Could you check a few things on this model? Use its own coordinates, in mm. Face numbers are marked on the shaded views. A direction names the side the tool comes from. Coordinates: 2 decimals unless noted, no trailing zeros. Loops run counter-clockwise (first coordinate to the right, second up) from the corner with the lowest first, then second, coordinate; pieces in that order, holes last. Notation, with made-up numbers: (-1.5, 12) - (41.5, 12) arc R15 ccw to (41.5, 37) - close; hole circle Ø7 at (9, 6.25). An arc over 180 degrees is marked (long way). Use CSV: the item, a comma, the result in double quotes.
from build123d import *

# Parameters (mm, degrees)
F0_W     = 50
F0_H     = 50
F1_DEPTH = 60
F4_DEPTH = 50.001
F5_DEPTH = 50.001


with BuildPart() as f1:
    # F0 (on Top) → F1 (new body)
    with BuildSketch(Plane.XY):
        with Locations((25, 25)):
            Rectangle(F0_W, F0_H)
    extrude(amount=F1_DEPTH)

    # F2 (on face) → F4 (intersect, through all)
    with BuildSketch(Plane.XZ):
        Polygon((50, 30), (25, 60), (0, 30), (25, 0), align=None)
        Polygon((25, 7.81025), (6.508541, 30), (25, 52.18975), (43.491459, 30), align=None, mode=Mode.SUBTRACT)
    extrude(amount=-F4_DEPTH, mode=Mode.INTERSECT)

    # F3 (on face) → F5 (intersect, through all)
    with BuildSketch(Plane(origin=(0, 0, 0), x_dir=(0, -1, 0), z_dir=(-1, 0, 0))):
        Polygon((-50, 30), (-25, 0), (0, 30), (-25, 60), align=None)
        Polygon((-6.508541, 30), (-25, 7.81025), (-43.491459, 30), (-25, 52.18975), align=None, mode=Mode.SUBTRACT)
    extrude(amount=-F5_DEPTH, mode=Mode.INTERSECT)


solid = f1.part
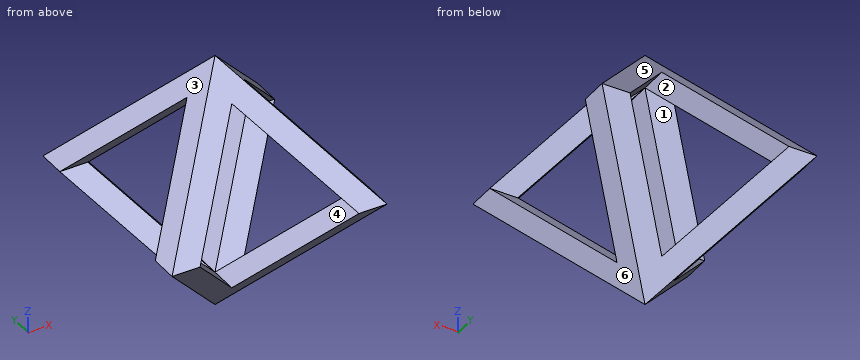
(1) Suppose I cut it at A-A (y = 10). Write out the boundary of the cut face in (x, z).
Computed:
outline,"(3.49, 25.81) - (10, 18) - (16.51, 18) - (10, 25.81) - close; (3.49, 34.19) - (10, 34.19) - (16.51, 42) - (10, 42) - close; (33.49, 18) - (40, 18) - (46.51, 25.81) - (40, 25.81) - close; (33.49, 42) - (40, 34.19) - (46.51, 34.19) - (40, 42) - close"
(2) Will these pins go through, and if not, where does the flat tip stop? pin 1 (1 mm diameter, centred on x = 11.5, y = 10, fed in from -Z); pin 2 (1 mm diameter, centred on x = 8.5, z = 40, fed in from +Y); pin 3 (2 mm diameter, centred on x = 42, y = 11, fed in from +Z); pin 4 (2 mm diameter, centred on x = 19.5, z = 43.5, fed in from -Y).
Computed:
pin 1,"stops at z = 17.4"
pin 2,"stops at y = 42.08"
pin 3,"stops at z = 40.8"
pin 4,"passes through"
(3) Please list where these lines run through material, in increasing order: line 1 (X direction, y = 34.5, z = 13.5); line 2 (Z direction, x = 16, y = 39); line 3 (Y direction, x = 38, z = 42).
Computed:
line 1,"x = 13.75 to 20.26, 29.74 to 36.25"
line 2,"z = 16.8 to 18.61, 41.39 to 43.2"
line 3,"y = 10 to 16.51, 33.49 to 40"
(4) Suppose I cut it at B-B (z = 42). Write out the boundary of the cut face in (x, y).
Computed:
outline,"(10, 10) - (16.51, 10) - (16.51, 16.51) - (10, 16.51) - close; (10, 33.49) - (16.51, 33.49) - (16.51, 40) - (10, 40) - close; (33.49, 10) - (40, 10) - (40, 16.51) - (33.49, 16.51) - close; (33.49, 33.49) - (40, 33.49) - (40, 40) - (33.49, 40) - close"
(5) Suppose I cut it at C-C (x = 5). Write out the boundary of the cut face in (y, z).
Computed:
outline,"(0, 30) - (5, 24) - (11.51, 24) - (6.51, 30) - (11.51, 36) - (5, 36) - close; (38.49, 24) - (45, 24) - (50, 30) - (45, 36) - (38.49, 36) - (43.49, 30) - close"
(6) Thinking about a two-plate mould opening in Z: for the marked faces 4, 5 and 6, which applies, +Z half, -Z half, draft (parallel to the pull), parting line (faces both ways), or undercut?
Computed:
face 4,"undercut"
face 5,"+Z half"
face 6,"-Z half"
(7) Which directions (+Z, -Z, +X, -X, +Y, -Y) give clear straight access to the entire face, cutting with the end or side of a thin tool? Please do the marked faces 1, 2 and 3.
Computed:
face 1,"+X, -X"
face 2,"+Y, -Y"
face 3,"+Z, -X, +Y, -Y"
(8) Suppose I cut it at D-D (x = 21.5). Write out the boundary of the cut face in (y, z), plus the area to 3 significant figures.
Computed:
outline,"(14.99, 12.01) - (21.5, 4.2) - (28.5, 4.2) - (35.01, 12.01) - (28.5, 12.01) - (25, 7.81) - (21.5, 12.01) - close; (14.99, 47.99) - (21.5, 47.99) - (25, 52.19) - (28.5, 47.99) - (35.01, 47.99) - (28.5, 55.8) - (21.5, 55.8) - close"
area,"182 mm²"
